Source: three-view drawing plus pictorial views. Frame: mm from the lowest corner of the part. A direction names the side the tool comes from. Round coordinates to 2 decimals unless told otherwise and drop trailing zeros. Loops run counter-clockwise (first coordinate to the right, second up) from the corner with the lowest first, then second, coordinate; pieces in that order, holes last. Notation, with made-up numbers: M 40.5,77 L 55.5,77 A21 cw 55.5,81 Z; hole C 3.5,-20.5 d11. An arc over 180 degrees is marked long. Return JSON: item names as keys, results as strings. Group by question number.
1) Section D-D (z = 63). Output: boundary loops of the cut face in (x, y), plus the area to 4 significant figures.
2) Section B-B (y = 6.5). Output: boundary loops of the cut face in (x, z).
3) Contact query for flat-ended pins moving along their axis: P1, Ø15, axis at x = 66, z = 20, coming from the -Y side; P2, Ø4, axis at x = 118, z = 49.5, coming from the -Y side; P3, Ø10, axis at y = 77, z = 57, coming from the -X side; P4, Ø12, axis at x = 127.5, z = 68, coming from the +Y side. Output: stop coordinate, or through.
4) Material intervals for line 1 (X direction, y = 46, z = 46); line 2 (Z direction, x = 13, y = 18); line 3 (Z direction, x = 91.5, y = 9.5), sorted ascending. Write a range as from..to.
5) Section A-A (x = 75). Output: boundary loops of the cut face in (y, z).
6) Access query for the marked faces 1, 2, 3 and 4. Directions: +Z, -Z, +X, -X, +Y, -Y. A direction counts if a zero-diameter tool reaches every point of the face in a straight line with its end or side. Return the directions, or none.
7) Section C-C (z = 32). Output: boundary loops of the cut face in (x, y), plus the area to 3 significant figures.
8) Mould query, pull axis X, two halves, no side actions, for the marked faces 5, 6 and 7. Classes: +X half, -X half, draft (parallel to the pull), parting line (faces both ways), or undercut.
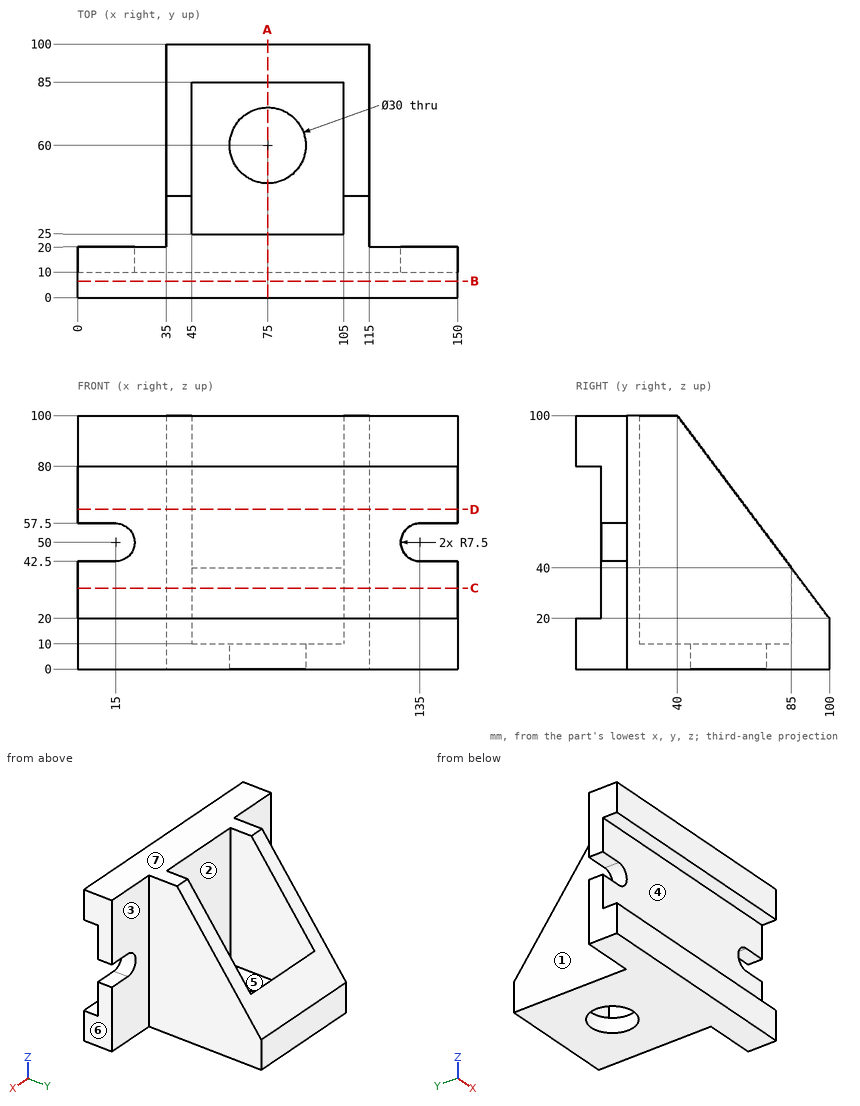
Returned:
{
 "1": {"outline": "M 0,10 L 150,10 L 150,20 L 115,20 L 115,67.75 L 105,67.75 L 105,25 L 45,25 L 45,67.75 L 35,67.75 L 35,20 L 0,20 Z", "area": "2,755 mm^2"},
 "2": {"outline": "M 0,0 L 150,0 L 150,20 L 0,20 Z; M 0,80 L 150,80 L 150,100 L 0,100 Z"},
 "3": {"P1": "stops at y = 0", "P2": "stops at y = 10", "P3": "stops at x = 35", "P4": "stops at y = 20"},
 "4": {"line 1": "x = 35..45, 105..115", "line 2": "z = 0..42.5, 57.5..100", "line 3": "z = 0..20, 80..100"},
 "5": {"outline": "M 0,0 L 45,0 L 45,10 L 25,10 L 25,100 L 0,100 L 0,80 L 10,80 L 10,20 L 0,20 Z; M 75,0 L 100,0 L 100,20 L 85,40 L 85,10 L 75,10 Z"},
 "6": {"face 1": "+Z, -Z, -X, +Y", "face 2": "+Z", "face 3": "+Z, -Z, +X, +Y", "face 4": "+X, -X, -Y"},
 "7": {"outline": "M 0,10 L 150,10 L 150,20 L 115,20 L 115,91 L 35,91 L 35,20 L 0,20 Z; hole M 45,25 L 105,25 L 105,85 L 45,85 Z", "area": "3,580 mm^2"},
 "8": {"face 5": "undercut", "face 6": "+X half", "face 7": "draft"}
}
